```python
from build123d import *

# Parameters (mm, degrees)
SKETCH_2_R          = 7
EXTRUDE_1_DEPTH     = 43
SKETCH_5_W          = 34
SKETCH_5_H          = 19
CUT_EXTRUDE_2_DEPTH = 35
SKETCH_6_W          = 62.498626105
SKETCH_6_H          = 38.983271372
CUT_EXTRUDE_3_DEPTH = 19
CUT_EXTRUDE_START   = -32
CUT_EXTRUDE_5_DEPTH = 24


with BuildPart() as part:
    # 草圖2 → 填料-伸長1 (new body)
    with BuildSketch(Plane.XY):
        with BuildLine():
            Line((-14, 11), (-14, -7))
            Line((-14, -7), (-7, -14))
            Line((-7, -14), (25.575538911, -14))
            ThreePointArc((25.575538911, -14), (28.840774692, -15.213413768), (30.521177653, -18.264705882))
            ThreePointArc((30.521177653, -18.264705882), (32.858007856, -26.115672061), (37.296980053, -33))
            Line((37.296980053, -33), (43, -33))
            Line((43, -33), (72, 1))
            Line((72, 1), (72, 20))
            Line((72, 20), (67, 25))
            Line((67, 25), (43, 25))
            ThreePointArc((43, 25), (34.561098706, 15.982044142), (22.361380836, 14.057085233))
            Line((22.361380836, 14.057085233), (0, 18))
            Line((0, 18), (-7, 18))
            Line((-7, 18), (-14, 11))
        make_face()
        Circle(SKETCH_2_R, mode=Mode.SUBTRACT)
    extrude(amount=EXTRUDE_1_DEPTH)

    # 草圖5 → 除料-伸長2 (cut, symmetric)
    with BuildSketch(Plane(origin=(0, 0, 0), x_dir=(1, 0, 0), z_dir=(0, 1, 0))):
        with Locations((3, -33.5)):
            Rectangle(SKETCH_5_W, SKETCH_5_H)
    extrude(amount=CUT_EXTRUDE_2_DEPTH, both=True, mode=Mode.SUBTRACT)

    # 草圖6 → 除料-伸長3 (cut)
    with BuildSketch(Plane.XY.offset(43)):
        with Locations((47.348473669, -33.491635686)):
            Rectangle(SKETCH_6_W, SKETCH_6_H)
    extrude(amount=-CUT_EXTRUDE_3_DEPTH, mode=Mode.SUBTRACT)

    # 草圖9 → 除料-伸長5 (cut)
    with BuildSketch(Plane.XY.offset(43).offset(CUT_EXTRUDE_START)):
        with BuildLine():
            ThreePointArc((33.236936549, 15.344294617), (44.184262982, -1.419294771), (61.764705882, -11))
            Line((61.764705882, -11), (72, 1))
            Line((72, 1), (72, 20))
            Line((72, 20), (67, 25))
            Line((67, 25), (43, 25))
            ThreePointArc((43, 25), (39.021244343, 19.259333621), (33.236936549, 15.344294617))
        make_face()
        with BuildLine():
            Line((72, 1), (61.764705882, -11))
            ThreePointArc((61.764705882, -11), (97.113272797, -3.706821839), (113, 28.701873436))
            ThreePointArc((113, 28.701873436), (65.22820561, 69.138772436), (33.236936549, 15.344294617))
            ThreePointArc((33.236936549, 15.344294617), (39.021244343, 19.259333621), (43, 25))
            Line((43, 25), (67, 25))
            Line((67, 25), (72, 20))
            Line((72, 20), (72, 1))
        make_face()
    extrude(amount=CUT_EXTRUDE_5_DEPTH, mode=Mode.SUBTRACT)


solid = part.part
```
Geometry: final body of the model. Coordinates: model frame, mm. A direction names the side the tool comes from. Give positions to 0.01 mm unless a question says otherwise; leave off trailing zeros. Write each loop counter-clockwise with the first axis right and the second up, starting at its lowest first coordinate (ties: lowest second). Pieces come first, ordered by that corner, then holes.
1. Draft query along X for faces 1 (the cylindrical face through (32.81, -26.01, 11.83)), 2 (the flat face through (55, 25, 5)), 3 (the cylindrical face through (6.466, -2.681, 11.832)). Return one class per face: released by +X, released by -X, zero draft, split by the parting line, or undercut.
2. Section query A-A, the plane z = 16.5. Return loops of the section in (x, y), then the cut area to 3 significant figures.
3. Section query B-B, the plane y = 6. Return loops of the section in (x, z).
4. Reachability of faces 4 (the flat face through (57.297, -16.238, 16.421)), 5 (the cylindrical face through (43.98, -1.23, 22.83)), 6 (the flat face through (-3, 18, 12)), 7 (the flat face through (20, 0, 34)), 8 (the flat face through (42, -21, 24)) from +Z, -Z, +X, -X, +Y, -Y: full face, straight path, thin tool, end or side. Return the list, or none.
5. Section query D-D, the plane z = 29.5. Return loops of the section in (x, y).
6. Section query C-C, the plane x = 41. Return loops of the section in (y, z), then the cut area to 3 significant figures.
7. Pin query (flat end, axial travel): P1, Ø1, axis at y = -2, z = 36, coming from the -X side; P2, Ø9.5, axis at x = -5, y = -4, coming from the +Z side; P3, Ø2, axis at x = -5, z = 11, coming from the +Y side. Return the tip coordinate at first contact, or that it passes through.
8. Line query: probe 1 along Y at (x, z) = (0, 11); probe 2 along Z at (x, y) = (50, 4); probe 3 along X at (y, z) = (0, 8.25). Output: solid intervals per line, ascending.
Computed:
1. face 1: released by -X
1. face 2: zero draft
1. face 3: undercut
2. outline: (-14, -7) - (-7, -14) - (25.58, -14) arc R5 cw to (30.52, -18.26) arc R29 ccw to (37.3, -33) - (43, -33) - (61.76, -11) arc R41 cw to (33.24, 15.34) arc R19 cw to (22.36, 14.06) - (0, 18) - (-7, 18) - (-14, 11) - close; hole circle Ø14 at (0, 0)
2. area: 1,910 mm2
3. outline: (-14, 0) - (-3.61, 0) - (-3.61, 24) - (-14, 24) - close; (3.61, 0) - (72, 0) - (72, 11) - (37.86, 11) - (37.86, 35) - (72, 35) - (72, 43) - (20, 43) - (20, 24) - (3.61, 24) - close
4. face 4: +Z, -Z, +X, -Y
4. face 5: +X, +Y
4. face 6: +Z, -Z, -X, +Y
4. face 7: +Z, -X, +Y, -Y
4. face 8: +Z, +X, -X, -Y
5. outline: (20, -14) - (59.21, -14) - (61.76, -11) arc R41 cw to (33.24, 15.34) arc R19 cw to (22.36, 14.06) - (20, 14.47) - close
6. outline: (-33, 0) - (21.56, 0) - (21.56, 11) - (1.87, 11) - (1.87, 35) - (21.56, 35) - (21.56, 43) - (-14, 43) - (-14, 24) - (-33, 24) - close
6. area: 1,510 mm2
7. P1: stops at x = 20
7. P2: stops at z = 24
7. P3: stops at y = 18
8. probe 1: y = -14 to -7, 7 to 18
8. probe 2: z = 0 to 11, 35 to 43
8. probe 3: x = -14 to -7, 7 to 71.15
